Geometry: final body of the model. Coordinates: model frame, mm. A direction names the side the tool comes from. Give positions to 0.01 mm unless a question says otherwise; leave off trailing zeros. Write each loop counter-clockwise with the first axis right and the second up, starting at its lowest first coordinate (ties: lowest second). Pieces come first, ordered by that corner, then holes. Notation, with made-up numbers: M 30,80.25 L 69,80.25 A30 cw 69,109.25 Z; hole C -17.5,-31.5 d3. An arc over 180 degrees is marked long. Use one line per item in the form item = value. Start each with the question number.
Item 1: Pull-direction query (X, two-part tool) for faces 1 (the cylindrical face through (27.003, -0.631, 0.592)), 2 (the cylindrical face through (17.535, -33.713, -1.726)), 3 (the flat face through (-1, 1, -3.5)); classes: released by +X, released by -X, zero draft, split by the parting line, or undercut.
Item 2: Section query C-C on z = 3. Return loops of the section in (x, y) (3 decimals).
Item 3: Access query for faces 4 (the cylindrical face through (-22.997, -0.631, 0.592)), 5 (the flat face through (17, -31, 0)). Directions: +Z, -Z, +X, -X, +Y, -Y. A direction counts if a zero-diameter tool reaches every point of the face in a straight line with its end or side. Return the directions, or none.
Item 4: Section query D-D on y = 25. Return loops of the section in (x, z), then the cut area to 3 significant figures.
Item 5: Section query A-A on y = 0. Return loops of the section in (x, z) (3 decimals), then the cut area to 3 significant figures.
Item 6: Contact query for flat-ended pins moving along their axis: P1, Ø6.5, axis at x = 25, y = 0, coming from the +Z side; P2, Ø3.5, axis at x = 0, y = -25, coming from the +Z side; P3, Ø1.5, axis at x = 13, z = 3, coming from the -Y side; P4, Ø3, axis at y = -18, z = 3.5, coming from the -X side. Output: stop coordinate, or through.
Item 7: Material intervals for line 1 along Y through (x, z) = (0, 1.25) (3 decimals); line 2 along X through (y, z) = (-24, 3.75); line 3 along Y through (x, z) = (-14, 3.5), sorted ascending. Write a range as from..to.
Autodesk Inventor part; units mm, degrees
ref_plane "YZ Plane" through (0, 0, 0) normal (1, 0, 0) x (0, 1, 0)
ref_plane "XZ Plane" through (0, 0, 0) normal (0, 1, 0) x (-1, 0, 0)
ref_plane "XY Plane" through (0, 0, 0) normal (0, 0, 1) x (1, 0, 0)
sketch "Sketch1" plane through (0, 0, 0) normal (0, 0, 1) x (1, 0, 0)
  circle A0 centre (0, 0) radius 34.925
  circle A1 centre (0, 0) radius 38
  circle A2 centre (-25, 0) radius 2.1
  circle A3 centre (0, -25) radius 2.1
  circle A4 centre (25, 0) radius 2.1
  circle A5 centre (0, 25) radius 2.1
  dimension "d0" = 69.85
  dimension "d1" = 76
  dimension "d6" = 25
  dimension "d7" = 4.2
  dimension "d10" = 360
extrude "Extrusion1" add sketch "Sketch1" along normal blind 4.8 contours A0
extrude "Extrusion2" add sketch "Sketch1" against normal blind 3.5 contours A0 | A1
properties part number "Fix_toDown_bearing" material "PLA Plastic"
Answer sheet:
q1.face_1 = undercut
q1.face_2 = split by the parting line
q1.face_3 = zero draft
q2.outline = C 0,0 d69.85; hole C -25,0 d4.2; hole C 0,-25 d4.2; hole C 0,25 d4.2; hole C 25,0 d4.2
q3.face_4 = +Z, -Z
q3.face_5 = +Z
q4.outline = M -28.62,-3.5 L -2.1,-3.5 L -2.1,4.8 L -24.39,4.8 L -24.39,0 L -28.62,0 Z; M 2.1,-3.5 L 28.62,-3.5 L 28.62,0 L 24.39,0 L 24.39,4.8 L 2.1,4.8 Z
q4.area = 400 mm2
q5.outline = M -38,-3.5 L -27.1,-3.5 L -27.1,4.8 L -34.925,4.8 L -34.925,0 L -38,0 Z; M -22.9,-3.5 L 22.9,-3.5 L 22.9,4.8 L -22.9,4.8 Z; M 27.1,-3.5 L 38,-3.5 L 38,0 L 34.925,0 L 34.925,4.8 L 27.1,4.8 Z
q5.area = 532 mm2
q6.P1 = 4.8
q6.P2 = through
q6.P3 = -32.71
q6.P4 = -30.78
q7.line_1 = -34.925..-27.1, -22.9..22.9, 27.1..34.925
q7.line_2 = -25.37..-1.85, 1.85..25.37
q7.line_3 = -32..32
